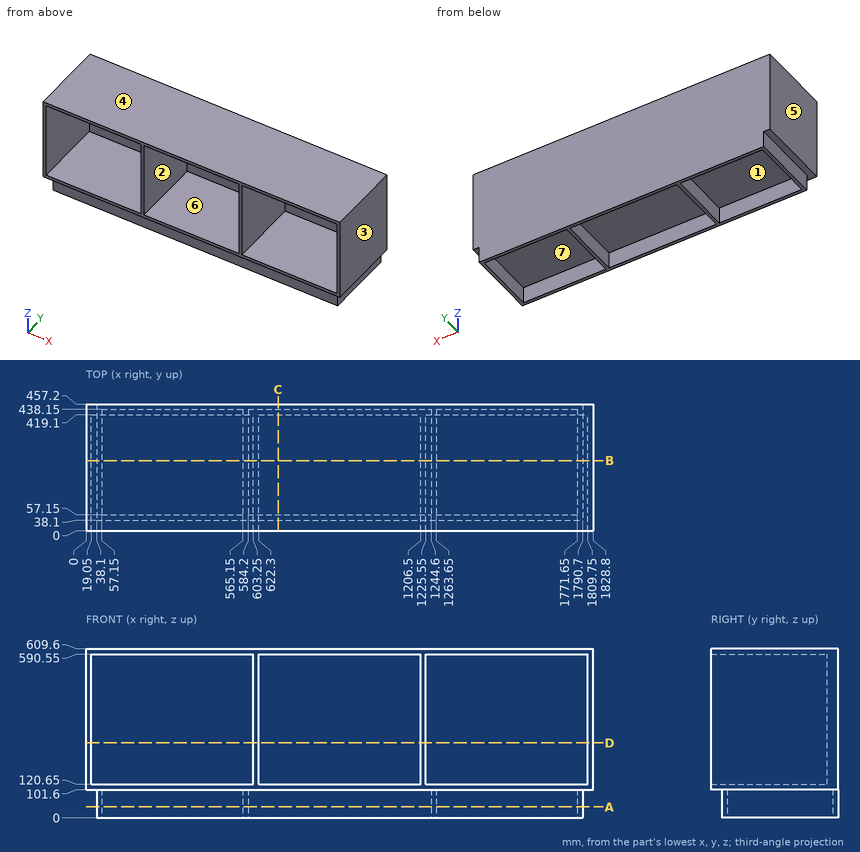
Geometry check sheet. Reference: drawing and pictorial views, mm from the part's lowest x, y, z. A direction names the side the tool comes from. Give positions to 0.01 mm unless a question says otherwise; leave off trailing zeros. Order: outer loops, then holes, each group sorted by start corner. A loop starts at its lowest first (then second) coordinate and runs counter-clockwise, first axis right, second up. Notation, with made-up numbers: M 71.5,63.25 L 101.5,63.25 A26 cw 101.5,92.25 Z; hole C 59.25,28 d9. An arc over 180 degrees is marked long. Answer as CSV lines item,"result". Start each with the question number.
Item 1: Tool access check on the marked faces 5, 6 and 7. Record the directions out of +Z, -Z, +X, -X, +Y, -Y that give a thin tool (end or side, any length) a straight path to the whole face; none if there is none.
Item 2: Thickness scan on line 1 (X direction, y = 149, z = 283); line 2 (Z direction, x = 1516.5, y = 106.5); line 3 (Y direction, x = 450, z = 60.5). Record the ranges inside material, lowest first. Write a range as [from, to].
Item 3: Mould release check, pull along Z, two halves, no side actions. Record for the marked faces 1, 2, 3 and 4: +Z half, -Z half, draft (parallel to the pull), parting line (faces both ways), or undercut.
Item 4: Cross-section at A-A on z = 40. Enter the section's corners in (x, y), plus the area to 3 significant figures.
Item 5: Cross-section at B-B on y = 253. State how many separate pieces and enclosed holes the cut face has, plus the area to 3 significant figures.
Item 6: Gauge pin test, flat ends, axial feed: P1, Ø8, axis at x = 506, z = 415.5, coming from the -Y side; P2, Ø1, axis at x = 1030, y = 177, coming from the -Z side. Record the tip position at first contact, or that the pin passes through.
Item 7: Cross-section at C-C on x = 693. Enter the section's corners in (y, z).
Item 8: Cross-section at D-D on z = 270. Enter the section's corners in (x, y).
Established:
1,face 5,"+Z, -Z, -X, +Y, -Y"
1,face 6,"-Y"
1,face 7,"-Z"
2,line 1,"x = [0, 19.05], [603.25, 622.3], [1206.5, 1225.55], [1809.75, 1828.8]"
2,line 2,"z = [101.6, 120.65], [590.55, 609.6]"
2,line 3,"y = [38.1, 57.15], [438.15, 457.2]"
3,face 1,"-Z half"
3,face 2,"undercut"
3,face 3,"draft"
3,face 4,"+Z half"
4,outline,"M 38.1,38.1 L 1790.7,38.1 L 1790.7,457.2 L 38.1,457.2 Z; hole M 57.15,57.15 L 565.15,57.15 L 565.15,438.15 L 57.15,438.15 Z; hole M 584.2,57.15 L 1244.6,57.15 L 1244.6,438.15 L 584.2,438.15 Z; hole M 1263.65,57.15 L 1771.65,57.15 L 1771.65,438.15 L 1263.65,438.15 Z"
4,area,"95,800 mm^2"
5,separate pieces,"1"
5,enclosed holes,"3"
5,area,"113,000 mm^2"
6,P1,"stops at y = 419.1"
6,P2,"stops at z = 101.6"
7,outline,"M 0,101.6 L 38.1,101.6 L 38.1,0 L 57.15,0 L 57.15,101.6 L 438.15,101.6 L 438.15,0 L 457.2,0 L 457.2,609.6 L 0,609.6 L 0,590.55 L 419.1,590.55 L 419.1,120.65 L 0,120.65 Z"
8,outline,"M 0,0 L 19.05,0 L 19.05,419.1 L 603.25,419.1 L 603.25,0 L 622.3,0 L 622.3,419.1 L 1206.5,419.1 L 1206.5,0 L 1225.55,0 L 1225.55,419.1 L 1809.75,419.1 L 1809.75,0 L 1828.8,0 L 1828.8,457.2 L 0,457.2 Z"
